The drawing under review shows one solid part. Ordinate dimensions are in mm from its lowest x, y, z. Round coordinates to 2 decimals unless told otherwise and drop trailing zeros. Order: outer loops, then holes, each group sorted by start corner. A loop starts at its lowest first (then second) coordinate and runs counter-clockwise, first axis right, second up. Notation, with made-up numbers: M 17.5,42 L 54.5,42 A13 ccw 54.5,55 Z; hole C 62,-26.75 d10. An arc over 180 degrees is marked long. Answer as a JSON object with one key per item and string values. Group by question number.
1) Consider section A-A, the plane y = 0.95. Write out the cut boundary in (x, z).
2) Consider section C-C, the plane x = 95. Write out the cut boundary in (y, z).
3) To check wall thickness, follow line 1 (X direction, y = 2.7, z = 25.5); line 2 (X direction, y = 0.75, z = 28.5); line 3 (X direction, y = 2.55, z = 30.5). State the ranges of each line that lie inside material, in increasing order.
4) Insertion check: pin 1 Ø2 at (x, y) = (250, 1.5) entering from -Z; pin 2 Ø2.5 at (x, z) = (192, 25) entering from -Y; pin 3 Ø2 at (x, y) = (224, 2.5) entering from +Z. Each pin has a flat end and moves straight along its axis. Give the tip position at first contact, or say it passes through.
5) Consider section B-B, the plane x = 14. Write out the cut boundary in (y, z), then the cut area to 3 significant figures.
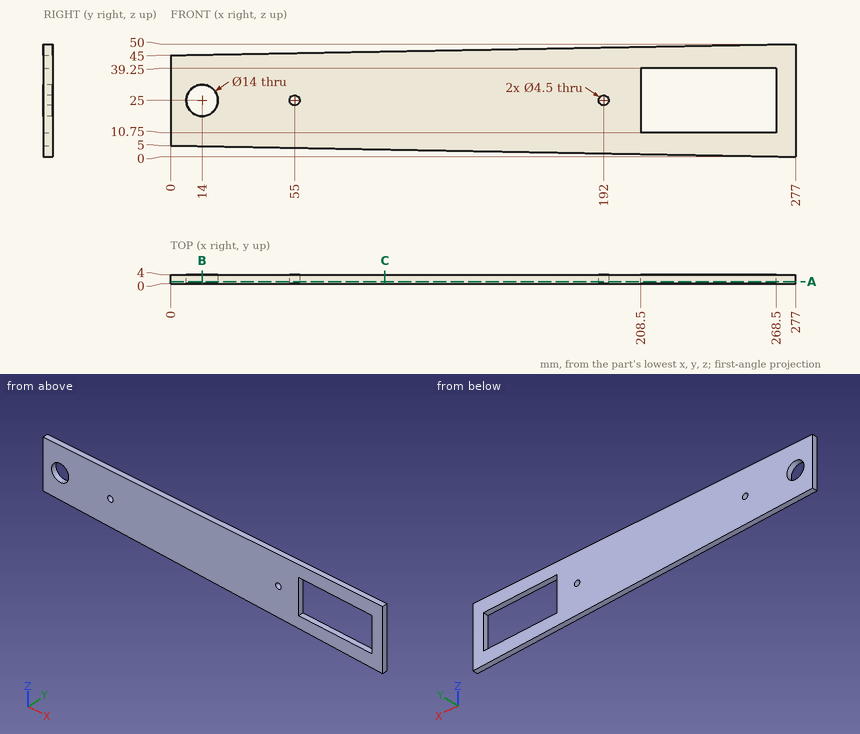
Results list:
{
 "1": {"outline": "M 0,5 L 277,0 L 277,50 L 0,45 Z; hole C 14,25 d14; hole C 55,25 d4.5; hole C 192,25 d4.5; hole M 208.5,10.75 L 268.5,10.75 L 268.5,39.25 L 208.5,39.25 Z"},
 "2": {"outline": "M 0,3.29 L 4,3.29 L 4,46.71 L 0,46.71 Z"},
 "3": {"line 1": "0 to 7.02, 20.98 to 52.81, 57.19 to 189.81, 194.19 to 208.5, 268.5 to 277", "line 2": "0 to 7.94, 20.06 to 208.5, 268.5 to 277", "line 3": "0 to 9.67, 18.33 to 208.5, 268.5 to 277"},
 "4": {"pin 1": "z = 0.47", "pin 2": "through", "pin 3": "z = 49.06"},
 "5": {"outline": "M 0,4.75 L 4,4.75 L 4,18 L 0,18 Z; M 0,32 L 4,32 L 4,45.25 L 0,45.25 Z", "area": "106 mm^2"}
}
